```python
from build123d import *

# Parameters (mm, degrees)
CHAMFER1_SIZE  = 1.27
SKETCH2_R      = 7.9375
EXTRUDE1_DEPTH = 11.1125
FILLET1_R      = 0.762
CHAMFER2_SIZE  = 0.762
FILLET2_R      = 0.762


with BuildPart() as part:
    # Sketch1 → Revolve1 (revolve)
    with BuildSketch(Plane.XY, mode=Mode.PRIVATE) as revolve1_sk:
        Polygon((127, 0), (127, 4.699), (113.03, 4.699), (113.03, 7.9375), (0, 7.9375), (0, 0), align=None)
    revolve(revolve1_sk.sketch.rotate(Axis((-72.566001994, 0, 0), (1, 0, 0)), 90), axis=Axis((-72.566001994, 0, 0), (1, 0, 0)))  # turned: the seam where the file's is

    # Chamfer1
    chamfer1_edges = [part.edges().sort_by_distance(p)[0] for p in [
        (127, 0, -4.699),
    ]]
    chamfer(chamfer1_edges, length=CHAMFER1_SIZE)

    # Sketch2 → Extrude1 (add)
    with BuildSketch(Plane.ZY):
        Polygon((5.953866916, -10.3124), (11.907733832, 0), (5.953866916, 10.3124), (-5.953866916, 10.3124), (-11.907733832, 0), (-5.953866916, -10.3124), align=None)
        Circle(SKETCH2_R, mode=Mode.SUBTRACT)
    extrude(amount=-EXTRUDE1_DEPTH)

    # Fillet1
    fillet1_edges = [part.edges().sort_by_distance(p)[0] for p in [
        (5.55625, -10.3124, 5.953866916),
        (5.55625, -10.3124, -5.953866916),
        (5.55625, 0, -11.907733832),
        (5.55625, 10.3124, -5.953866916),
        (5.55625, 10.3124, 5.953866916),
        (5.55625, 0, 11.907733832),
    ]]
    fillet(fillet1_edges, radius=FILLET1_R)

    # Chamfer2
    chamfer2_edges = [part.edges().sort_by_distance(p)[0] for p in [
        (113.03, 0, -7.9375),
    ]]
    chamfer(chamfer2_edges, length=CHAMFER2_SIZE)

    # Fillet2
    fillet2_edges = [part.edges().sort_by_distance(p)[0] for p in [
        (11.1125, 0, -7.9375),
    ]]
    fillet(fillet2_edges, radius=FILLET2_R)


solid = part.part
```
Verification items for the finished model (mm, model axes). A direction names the side the tool comes from. Coordinates: 2 decimals unless noted, no trailing zeros. Write each loop counter-clockwise with the first axis right and the second up, starting at its lowest first coordinate (ties: lowest second). Pieces come first, ordered by that corner, then holes. Notation, with made-up numbers: M 59.25,12 L 93.25,12 A18 ccw 93.25,27 Z; hole C 46,17 d10. An arc over 180 degrees is marked long. Answer as a JSON object with one key per item and string values. Group by question number.
(1) Cross-section at B-B, the plane x = 107. Record the cut outline in (y, z) (1 decimal).
(2) Cross-section at A-A, the plane z = 0. Record the cut outline in (x, y), and give its area (3 significant figures).
(3) Gauge pin test, flat ends, axial feed: pin 1 (3 mm diameter, centred on x = 86.5, y = 2, fed in from -Z); pin 2 (8 mm diameter, centred on x = 86, z = -3, fed in from +Y); pin 3 (1 mm diameter, centred on x = 78.5, z = -1, fed in from -Y); pin 4 (3 mm diameter, centred on x = 26.5, z = -9.5, fed in from +Y). Record the tip position at first contact, or that the pin passes through.
(4) Release check for a two-part mould opening along X. For faces 3 (the face through (5.478, 5.223, -8.892)), 4 (the face through (11.112, 4, -8)), 5 (the face through (0, 0, 0)) record: +X half, -X half, draft (parallel to the pull), parting line (faces both ways), or undercut.
(5) Material ranges on line 1 (Y direction, x = 43.5, z = -0.5); line 2 (Z direction, x = 70, y = 0.25); line 3 (X direction, y = -8, z = 3.5), recorded low to high.
(6) Tool access check on faces 1 (the face through (113.03, 1, -5)), 2 (the face through (5.478, -5.223, 8.892)). Record the directions out of +Z, -Z, +X, -X, +Y, -Y that give a thin tool (end or side, any length) a straight path to the whole face; none if there is none.
Reply:
{
 "1": {"outline": "C 0,0 d15.9"},
 "2": {"outline": "M 0,-10.31 L 11.11,-10.31 L 11.11,-8.7 A0.76 cw 11.87,-7.94 L 112.27,-7.94 L 113.03,-7.18 L 113.03,-4.7 L 125.73,-4.7 L 127,-3.43 L 127,3.43 L 125.73,4.7 L 113.03,4.7 L 113.03,7.18 L 112.27,7.94 L 11.87,7.94 A0.76 cw 11.11,8.7 L 11.11,10.31 L 0,10.31 Z", "area": "1,980 mm²"},
 "3": {"pin 1": "z = -7.92", "pin 2": "y = 7.94", "pin 3": "y = -7.92", "pin 4": "through"},
 "4": {"face 3": "draft", "face 4": "+X half", "face 5": "-X half"},
 "5": {"line 1": "-7.92 to 7.92", "line 2": "-7.93 to 7.93", "line 3": "0 to 11.11"},
 "6": {"face 1": "+X", "face 2": "+Z, +X, -X, -Y"}
}
